Geometry check sheet. Reference: the model listing, model coordinates, mm. A direction names the side the tool comes from. Round coordinates to 2 decimals unless told otherwise and drop trailing zeros. Order: outer loops, then holes, each group sorted by start corner. A loop starts at its lowest first (then second) coordinate and runs counter-clockwise, first axis right, second up. Notation, with made-up numbers: (84.25, 45) - (101.25, 45) arc R30 cw to (101.25, 67) - close; hole circle Ø9 at (-21.5, 57). An arc over 180 degrees is marked (long way). Use a Markdown table: item, result. Add a question column.
(1) Section check B-B on y = 23. Record the boundary of the cut face in (x, z), then the cut area to 3 significant figures.
(2) Section check C-C on y = 124.5. Record the boundary of the cut face in (x, z).
(3) Access from +Z, -Z, +X, -X, +Y, -Y to the whole of each face (thin tool, end or side, straight path). Record for faces 1 (the face through (-24.1, 57.4, 10)), 2 (the face through (-13.56, 130, 92)), 3 (the face through (-39, 33, 97)), 4 (the face through (-9.152, 114.416, 4.93)), 5 (the face through (-1, -34, 48)).
(4) Gauge pin test, flat ends, axial feed: P1, Ø4, axis at x = 35, y = 49, coming from the -Z side; P2, Ø1, axis at x = -62.5, y = -14, coming from the +Z side; P3, Ø5, axis at y = 132, z = 93, coming from the -X side; P4, Ø5, axis at x = -58, z = 10, coming from the +Y side. Record the tip position at first contact, or that the pin passes through.
(5) Thickness scan on line 1 along Y through (x, z) = (70.5, 70.5); line 2 along X through (y, z) = (69.5, 6.5); line 3 along Y through (x, z) = (-47, 6.5). Record the ranges inside material, lowest first. Write a range as [from, to].
(6) Mould release check, pull along X, two halves, no side actions. Record for faces 6 (the face through (-39, 33, 0)), 7 (the face through (-9.152, 114.416, 91.93)), 8 (the face through (-1, -24, 48)): released by +X, released by -X, zero draft, split by the parting line, or undercut.
(7) Section check D-D on z = 80. Record the boundary of the cut face in (x, y).
(8) Section check A-A on x = -40.5. Record the boundary of the cut face in (y, z), then the cut area to 3 significant figures.
```python
from build123d import *

# Parameters (mm, degrees)
F1_DEPTH = 97
F2_DEPTH = 87
F3_DEPTH = 10


with BuildPart() as f1:
    # F0 (on Top) → F1 (new body)
    with BuildSketch(Plane.XY):
        Polygon((-4.618802, 106.564065), (-80, -24), (-70.762396, -24), (-66.143594, -16), (0, 98.564065), (66.143594, -16), (70.762396, -24), (80, -24), (0, 114.564065), (-13.559861, 138.050432), (-13.559861, 122.050432), align=None)
        Polygon((-70.762396, -24), (-80, -24), (-85.773503, -34), (85.773503, -34), (80, -24), (70.762396, -24), align=None)
    extrude(amount=F1_DEPTH)

    # F0 (on Top) → F2 (cut)
    with BuildSketch(Plane.XY):
        Polygon((-4.618802, 106.564065), (-80, -24), (-70.762396, -24), (-66.143594, -16), (0, 98.564065), (66.143594, -16), (70.762396, -24), (80, -24), (0, 114.564065), (-13.559861, 138.050432), (-13.559861, 122.050432), align=None)
    extrude(amount=F2_DEPTH, mode=Mode.SUBTRACT)

    # F0 (on Top) → F3 (join)
    with BuildSketch(Plane.XY):
        Polygon((-4.618802, 106.564065), (-80, -24), (-70.762396, -24), (-66.143594, -16), (0, 98.564065), (66.143594, -16), (70.762396, -24), (80, -24), (0, 114.564065), (-13.559861, 138.050432), (-13.559861, 122.050432), align=None)
    extrude(amount=F3_DEPTH)


solid = f1.part
```
Check sheet entries:
| question | item | result |
|---|---|---|
| 1 | outline | (-52.86, 0) - (-43.63, 0) - (-43.63, 10) - (-52.86, 10) - close; (-52.86, 87) - (-43.63, 87) - (-43.63, 97) - (-52.86, 97) - close; (43.63, 0) - (52.86, 0) - (52.86, 10) - (43.63, 10) - close; (43.63, 87) - (52.86, 87) - (52.86, 97) - (43.63, 97) - close |
| 1 | area | 370 mm2 |
| 2 | outline | (-13.56, 0) - (-5.74, 0) - (-5.74, 10) - (-13.56, 10) - close; (-13.56, 87) - (-5.74, 87) - (-5.74, 97) - (-13.56, 97) - close |
| 3 | face 1 | +X, -X, +Y |
| 3 | face 2 | +Z, -Z, -X, +Y |
| 3 | face 3 | +Z, +X, -X, +Y, -Y |
| 3 | face 4 | +Z, -Z, -X |
| 3 | face 5 | +Z, -Z, +X, -X, -Y |
| 4 | P1 | stops at z = 0 |
| 4 | P2 | passes through |
| 4 | P3 | stops at x = -13.56 |
| 4 | P4 | stops at y = 18.44 |
| 5 | line 1 | y = [-34, -24] |
| 5 | line 2 | x = [-26.02, -16.78], [16.78, 26.02] |
| 5 | line 3 | y = [-34, -24], [17.16, 33.16] |
| 6 | face 6 | zero draft |
| 6 | face 7 | released by -X |
| 6 | face 8 | undercut |
| 7 | outline | (-85.77, -34) - (85.77, -34) - (80, -24) - (-80, -24) - close |
| 8 | outline | (-34, 0) - (-24, 0) - (-24, 97) - (-34, 97) - close; (28.42, 0) - (44.42, 0) - (44.42, 10) - (28.42, 10) - close; (28.42, 87) - (44.42, 87) - (44.42, 97) - (28.42, 97) - close |
| 8 | area | 1,290 mm2 |
